Can you work these out from the drawing? Everything is in mm from the part's minimum corner. Give positions to 0.01 mm unless a question says otherwise; leave off trailing zeros. Order: outer loops, then holes, each group sorted by start corner. A loop starts at its lowest first (then second) coordinate and runs counter-clockwise, first axis right, second up. Notation, with made-up numbers: (69, 32) - (84, 32) arc R13 cw to (84, 56) - close; hole circle Ø7 at (67, 23). An arc over 180 degrees is marked (long way). One line per question, with ' | ' between items.
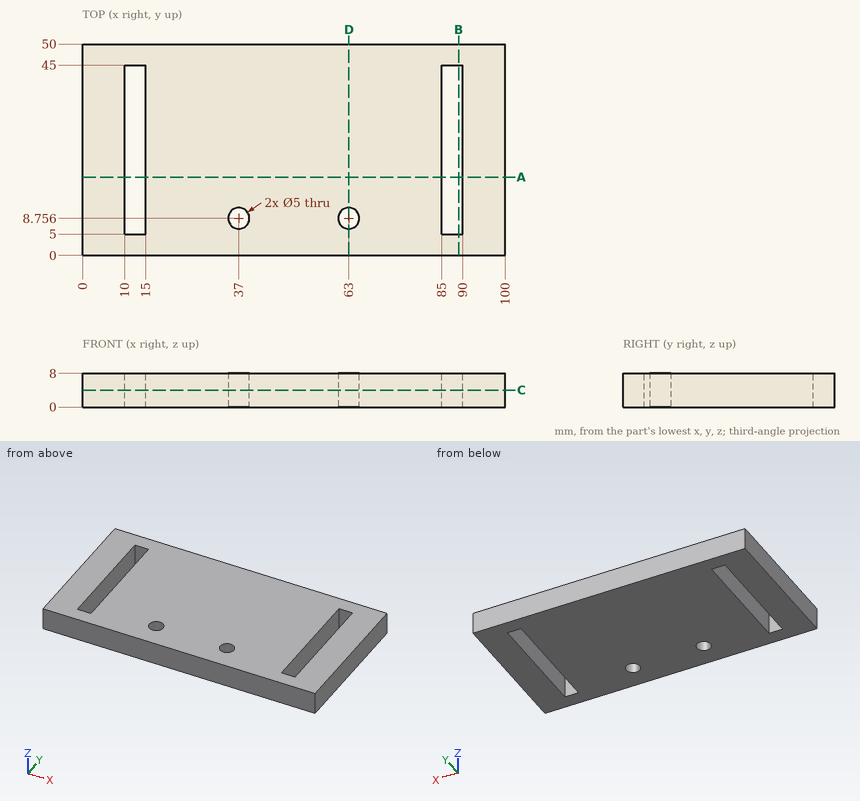
1) I want a section at D-D (x = 63). List the corners of the cut face in (y, z) for me.
Model answer:
outline: (0, 0) - (6.26, 0) - (6.26, 8) - (0, 8) - close; (11.26, 0) - (50, 0) - (50, 8) - (11.26, 8) - close
2) Please list where these lines run through material, in increasing order: L1, parallel to X at y = 9, z = 4.75; L2, parallel to X at y = 18.5, z = 1.25; L3, parallel to Y at x = 13, z = 1.5.
Model answer:
L1: x = 0 to 10, 15 to 34.51, 39.49 to 60.51, 65.49 to 85, 90 to 100 | L2: x = 0 to 10, 15 to 85, 90 to 100 | L3: y = 0 to 5, 45 to 50
3) I want a section at A-A (y = 18.5). List the corners of the cut face in (x, z) for me, plus the area to 3 significant figures.
Model answer:
outline: (0, 0) - (10, 0) - (10, 8) - (0, 8) - close; (15, 0) - (85, 0) - (85, 8) - (15, 8) - close; (90, 0) - (100, 0) - (100, 8) - (90, 8) - close | area: 720 mm2
4) I want a section at C-C (z = 4). List the corners of the cut face in (x, y) for me.
Model answer:
outline: (0, 0) - (100, 0) - (100, 50) - (0, 50) - close; hole (10, 5) - (15, 5) - (15, 45) - (10, 45) - close; hole circle Ø5 at (37, 8.76); hole circle Ø5 at (63, 8.76); hole (85, 5) - (90, 5) - (90, 45) - (85, 45) - close
5) I want a section at B-B (x = 89). List the corners of the cut face in (y, z) for me.
Model answer:
outline: (0, 0) - (5, 0) - (5, 8) - (0, 8) - close; (45, 0) - (50, 0) - (50, 8) - (45, 8) - close
